Part print with two shaded views. Sizes in mm from the minimum x, y, z corner. A direction names the side the tool comes from. Give positions to 0.01 mm unless a question says otherwise; leave off trailing zeros. Write each loop counter-clockwise with the first axis right and the second up, starting at its lowest first coordinate (ties: lowest second). Pieces come first, ordered by that corner, then holes. Notation, with made-up numbers: M -37,-38.5 L 4,-38.5 A28 ccw 4,-15.5 Z; hole C -1.75,74 d7. An arc over 180 degrees is marked long. Return JSON: item names as keys, results as strings. Group by question number.
Q1. Wall check: probe 1 along Z at (x, y) = (46.5, 114); probe 2 along X at (y, z) = (24.5, 57); probe 3 along Y at (x, z) = (73, 139.5). Give the ranges that are in metal, low to high.
Q2. Band-saw the part on B-B, the plane z = 134. Give the cut face in (x, y).
Q3. Flat gauge pins, fed straight in: pin 1 Ø12 at (x, z) = (74, 120) entering from -Y; pin 2 Ø10 at (x, z) = (38.5, 24.5) entering from +Y; pin 3 Ø12 at (y, z) = (83.5, 17.5) entering from -X; pin 4 Ø5 at (x, y) = (188.5, 100) entering from -Z. Where does each tip first touch, or does it go through?
Q4. Band-saw the part on A-A, the plane x = 115. Give the cut face in (y, z), then the cut area to 3 significant figures.
Q5. Tool access for the marked faces 1 and 2: list every direction of +Z, -Z, +X, -X, +Y, -Y with a clear straight run to the whole face (end or side of a thin tool).
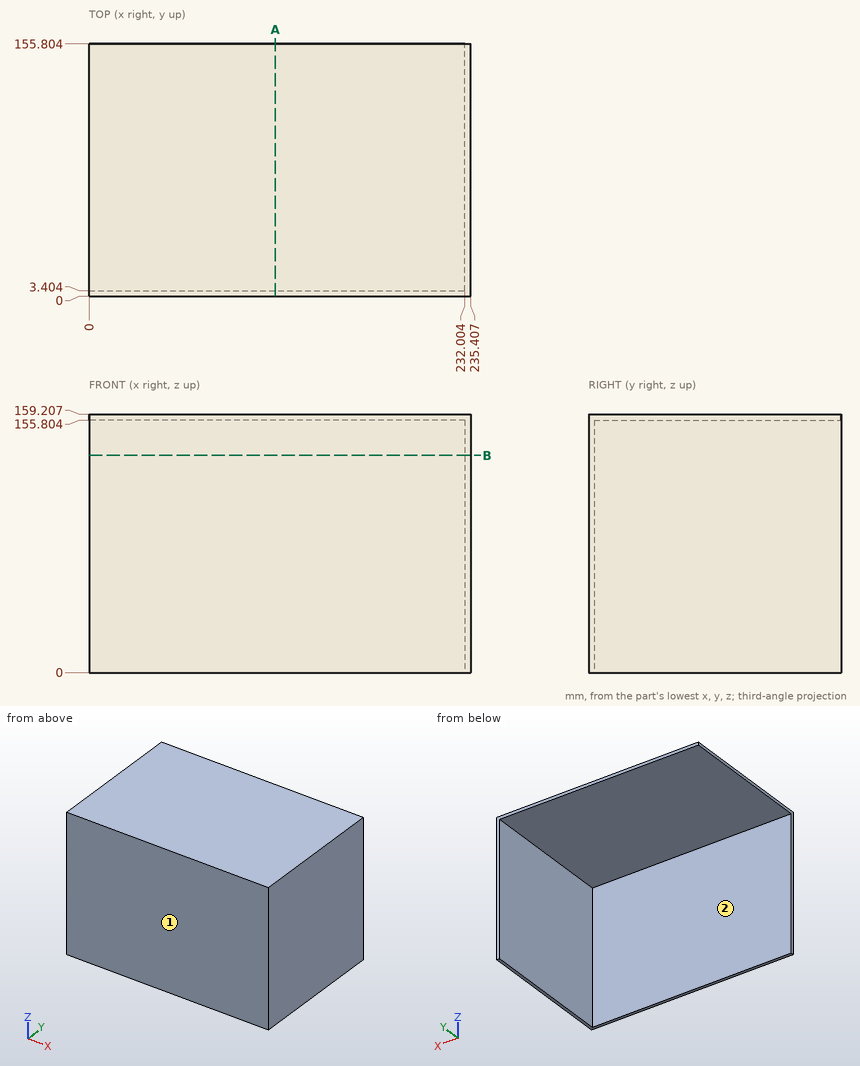
From the geometry:
{
 "1": {"probe 1": "z = 155.8 to 159.21", "probe 2": "x = 232 to 235.41", "probe 3": "y = 0 to 3.4"},
 "2": {"outline": "M 0,0 L 235.41,0 L 235.41,155.8 L 232,155.8 L 232,3.4 L 0,3.4 Z"},
 "3": {"pin 1": "stops at y = 0", "pin 2": "stops at y = 3.4", "pin 3": "stops at x = 232", "pin 4": "stops at z = 155.8"},
 "4": {"outline": "M 0,0 L 3.4,0 L 3.4,155.8 L 155.8,155.8 L 155.8,159.21 L 0,159.21 Z", "area": "1,060 mm^2"},
 "5": {"face 1": "+Z, -Z, +X, -X, -Y", "face 2": "-Z, -X, +Y"}
}
